Work out the finished part from the listing and answer in its coordinate system (mm). A direction names the side the tool comes from. Coordinates: 2 decimals unless noted, no trailing zeros. Order: outer loops, then holes, each group sorted by start corner. A loop starts at its lowest first (then second) coordinate and runs counter-clockwise, first axis right, second up. Notation, with made-up numbers: (40, 8) -> (99, 8) arc R9 ccw to (99, 25) -> close; hole circle Ø6 at (8.25, 34.5). An arc over 180 degrees is marked (long way). Write item = value, one per line. Start each with the question number.
Q1. The part is cut by section C-C, the plane z = 2. Determine the outline of the cut face in (x, y) (3 decimals).
Q2. Straight lines are drawn through the part: L1, parallel to Z at x = -116, y = 51.5; L2, parallel to Y at x = -115.5, z = 4.5; L3, parallel to X at y = 55, z = 15. For each, find the intervals that lie inside material, in ascending order. Write a range as from..to.
Q3. Which of the six approach directions +Z, -Z, +X, -X, +Y, -Y give full straight-line access (tool end or side, diameter ignored) to faces 4 (the flat face through (-115, 53, 0)), 5 (the flat face through (-115, 53, 1.27))?
Q4. Flat-ended cylindrical pins translate along their axes: pin 1 (8.5 mm diameter, centred on x = -115.5, y = 55, fed in from +Z); pin 2 (1 mm diameter, centred on y = 53.5, z = 11, fed in from +X); pin 3 (3 mm diameter, centred on y = 58.5, z = 4, fed in from -X). Find the tip coordinate at first contact, or state that the pin passes through.
Q5. The part is cut by section B-B, the plane x = -108.5. Determine the outline of the cut face in (y, z) (3 decimals), plus the area to 3 significant figures.
Q6. For a pull along Y with two mould halves and no side action, classify faces 1 (the cylindrical face through (-106.057, 55.483, 9.392)), 2 (the flat face through (-115.2, 61.1, 19.05)), 3 (the cylindrical face through (-121.693, 47.599, 10.036)) as +Y half, -Y half, draft (parallel to the pull), parting line (faces both ways), or undercut.
Q7. The part is cut by section A-A, the plane x = -116.25. Determine the outline of the cut face in (y, z).
```python
from build123d import *

# Parameters (mm, degrees)
F0_R     = 9.525
F1_DEPTH = 19.05
F2_T     = -1.27
F4_D     = 0.635


# Not quite as in the source:
# - the program builds the solid bodies; features that only make, move or delete a surface that nothing else refers to are left out


with BuildPart() as f1:
    # F0 (on Top) → F1 (new body)
    with BuildSketch(Plane.XY):
        with Locations((-115.1416823268, 52.6224188507)):
            Circle(F0_R)
    extrude(amount=F1_DEPTH)

    # F2
    f2_openings = [f1.faces().sort_by_distance(p)[0] for p in [
        (-115.141682, 52.622419, 19.05),
    ]]
    offset(amount=F2_T, openings=f2_openings)

    # F4 (through all)
    with Locations(Plane.XY.offset(1.27)):
        with Locations((-116.9411316514, 59.9756650627), (-114.9873510003, 58.9685030282), (-113.8059347868, 58.9685030282), (-117.4980401993, 58.4304407239), (-119.3492934108, 57.1395158768), (-121.0996806622, 55.9318587184), (-119.9708729982, 54.7268129885), (-116.9627532363, 57.0406801999), (-116.2916645408, 56.6788762808), (-117.056325078, 55.0978146493), (-118.0468276143, 53.8730248809), (-120.9187433124, 52.0108155906), (-120.5618828535, 51.0843060911), (-118.0632561445, 51.9599355757), (-118.6012327671, 48.8700121641), (-117.4913495779, 49.2096692324), (-115.4741570354, 50.8750453591), (-115.1792779565, 53.5607412457), (-114.4042313099, 57.1855939925), (-113.5956719518, 55.5465482175), (-111.127205193, 57.0756867528), (-110.8181774616, 56.6184930503), (-112.3543679714, 54.7396689653), (-111.7949485779, 52.8271049261), (-110.0980043411, 54.0584772825), (-110.5114147067, 51.1053167284), (-113.6578395963, 51.2212850153), (-114.1850054264, 49.5988503098), (-112.0592430234, 48.9115975797), (-115.2876019478, 47.3995991051), (-112.5525608659, 57.9002201557)):
            Hole(F4_D / 2)


solid = f1.part
```
Model answer:
q1.outline = circle Ø19.05 at (-115.142, 52.622); hole circle Ø16.51 at (-115.142, 52.622)
q2.L1 = 0..1.27
q2.L2 = 43.1..44.38, 60.87..62.14
q2.L3 = -124.37..-123.05, -107.24..-105.92
q3.face_4 = -Z, +X, -X, +Y, -Y
q3.face_5 = +Z
q4.pin_1 = 1.27
q4.pin_2 = -105.62
q4.pin_3 = -123.6
q5.outline = (45.795, 0) -> (59.45, 0) -> (59.45, 19.05) -> (57.525, 19.05) -> (57.525, 1.27) -> (47.72, 1.27) -> (47.72, 19.05) -> (45.795, 19.05) -> close
q5.area = 85.8 mm2
q6.face_1 = parting line
q6.face_2 = draft
q6.face_3 = undercut
q7.outline = (43.16, 0) -> (56.36, 0) -> (56.36, 1.27) -> (44.44, 1.27) -> (44.44, 19.05) -> (43.16, 19.05) -> close; (56.99, 0) -> (62.08, 0) -> (62.08, 19.05) -> (60.8, 19.05) -> (60.8, 1.27) -> (56.99, 1.27) -> close
